Autodesk Inventor part; units mm, degrees
ref_plane "YZ Plane" through (0, 0, 0) normal (1, 0, 0) x (0, 1, 0)
ref_plane "XZ Plane" through (0, 0, 0) normal (0, 1, 0) x (-1, 0, 0)
ref_plane "XY Plane" through (0, 0, 0) normal (0, 0, 1) x (1, 0, 0)
sketch "Sketch1" plane through (0, 0, 0) normal (1, 0, 0) x (0, 1, 0)
  line L0 (0, 0) -> (0, -3.9878)
  line L1 (0, -3.9878) -> (0, -6.35)
  line L2 (0, -6.35) -> (3.175, -6.35)
  line L3 (3.175, -6.35) -> (3.175, -3.9878)
  line L4 (9.525, -3.9878) -> (9.525, -6.35)
  line L5 (9.525, -6.35) -> (12.7, -6.35)
  line L6 (12.7, -6.35) -> (12.7, -3.9878)
  line L7 (19.05, -3.9878) -> (19.05, -6.35)
  line L8 (19.05, -6.35) -> (22.225, -6.35)
  line L9 (22.225, -6.35) -> (22.225, -3.9878)
  line L10 (25.7937, 0) -> (0, 0)
  line L11 (51.5874, 0) -> (51.5874, -3.175)
  line L12 (51.5874, -3.175) -> (51.5874, -6.35)
  line L13 (51.5874, -6.35) -> (48.4124, -6.35)
  line L14 (48.4124, -6.35) -> (48.4124, -3.9878)
  line L15 (42.0624, -3.9878) -> (42.0624, -6.35)
  line L16 (42.0624, -6.35) -> (38.8874, -6.35)
  line L17 (38.8874, -6.35) -> (38.8874, -3.9878)
  line L18 (32.5374, -3.9878) -> (32.5374, -6.35)
  line L19 (32.5374, -6.35) -> (29.3624, -6.35)
  line L20 (29.3624, -6.35) -> (29.3624, -3.9878)
  line L21 (25.7937, 0) -> (51.5874, 0)
  line L22 (3.175, -3.9878) -> (9.525, -3.9878)
  line L23 (12.7, -3.9878) -> (19.05, -3.9878)
  line L24 (22.225, -3.9878) -> (29.3624, -3.9878)
  line L25 (32.5374, -3.9878) -> (38.8874, -3.9878)
  line L26 (42.0624, -3.9878) -> (48.4124, -3.9878)
  dimension "d1" = 3.9878
  dimension "d2" = 2.3622
  dimension "d3" = 3.175
  dimension "d5" = 3.175
  dimension "d7" = 3.175
revolve "Revolution1" add sketch "Sketch1" angle 360 about axis through (0, 25.7937, 0) along (0, 1, 0)
properties part number "Crankshaft Crank Cylinder"
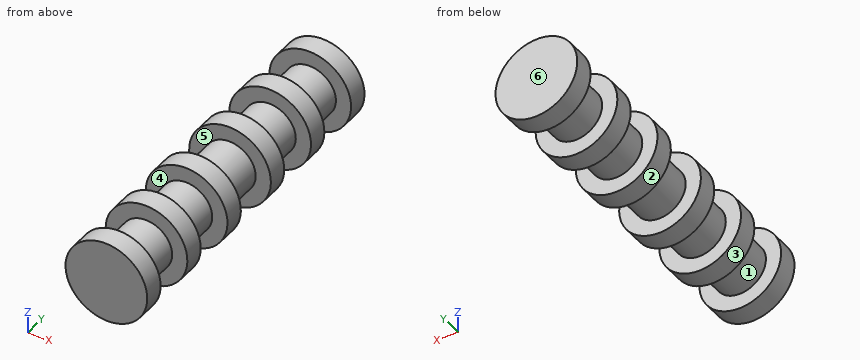
Verification items for the finished model (mm, model axes). Face numbers are marked on the shaded views. A direction names the side the tool comes from. Coordinates: 2 decimals unless noted, no trailing zeros. Loops run counter-clockwise (first coordinate to the right, second up) from the corner with the lowest first, then second, coordinate; pieces in that order, holes last. Notation, with made-up numbers: (87, -22.75) -> (138, -22.75) arc R7 cw to (138, -18.75) -> close; hole circle Ø11 at (19.5, 15.25). An arc over 180 degrees is marked (long way). Answer as CSV lines item,"result".
1) Tool access check on the marked faces 1 and 2. Record the directions out of +Z, -Z, +X, -X, +Y, -Y that give a thin tool (end or side, any length) a straight path to the whole face; none if there is none.
Found:
face 1,"none"
face 2,"+Y, -Y"
2) Depth check by flat-ended pin: pin 1 (1.5 mm diameter, centred on x = 2, y = 38.5, fed in from -Z); pin 2 (1.5 mm diameter, centred on y = 30, z = -4, fed in from +X); pin 3 (1.5 mm diameter, centred on x = -1.5, y = 24, fed in from -Z). Enter the tip coordinate at first touch or a pass-through.
Found:
pin 1,"stops at z = -6.2"
pin 2,"stops at x = 5.46"
pin 3,"stops at z = -3.92"
3) Thickness scan on L1, parallel to Y at x = 4, z = -1 (3 decimals); L2, parallel to Z at x = 0, y = 27; L3, parallel to Z at x = 1.75, y = 35. Record the ranges inside material, lowest first. Write a range as from..to.
Found:
L1,"y = 0..3.175, 9.525..12.7, 19.05..22.225, 29.362..32.537, 38.887..42.062, 48.412..51.587"
L2,"z = -3.99..3.99"
L3,"z = -3.58..3.58"
4) Cross-section at B-B, the plane z = -4.75. Record the cut outline in (x, y) (3 decimals), then the cut area to 3 significant figures.
Found:
outline,"(-4.214, 0) -> (4.214, 0) -> (4.214, 3.175) -> (-4.214, 3.175) -> close; (-4.214, 9.525) -> (4.214, 9.525) -> (4.214, 12.7) -> (-4.214, 12.7) -> close; (-4.214, 19.05) -> (4.214, 19.05) -> (4.214, 22.225) -> (-4.214, 22.225) -> close; (-4.214, 29.362) -> (4.214, 29.362) -> (4.214, 32.537) -> (-4.214, 32.537) -> close; (-4.214, 38.887) -> (4.214, 38.887) -> (4.214, 42.062) -> (-4.214, 42.062) -> close; (-4.214, 48.412) -> (4.214, 48.412) -> (4.214, 51.587) -> (-4.214, 51.587) -> close"
area,"161 mm2"
5) Cross-section at D-D, the plane y = 11.5. Record the cut outline in (x, z), then the cut area to 3 significant figures.
Found:
outline,"circle Ø12.7 at (0, 0)"
area,"127 mm2"
6) Cross-section at C-C, the plane y = 44. Record the cut outline in (x, z), then the cut area to 3 significant figures.
Found:
outline,"circle Ø7.98 at (0, 0)"
area,"50.0 mm2"
7) Release check for a two-part mould opening along Y. For the marked faces 3, 4, 5 and 6 record: +Y half, -Y half, draft (parallel to the pull), parting line (faces both ways), or undercut.
Found:
face 3,"draft"
face 4,"undercut"
face 5,"undercut"
face 6,"+Y half"
8) Cross-section at A-A, the plane x = -4.5. Record the cut outline in (y, z) (3 decimals).
Found:
outline,"(0, -4.48) -> (3.175, -4.48) -> (3.175, 4.48) -> (0, 4.48) -> close; (9.525, -4.48) -> (12.7, -4.48) -> (12.7, 4.48) -> (9.525, 4.48) -> close; (19.05, -4.48) -> (22.225, -4.48) -> (22.225, 4.48) -> (19.05, 4.48) -> close; (29.362, -4.48) -> (32.537, -4.48) -> (32.537, 4.48) -> (29.362, 4.48) -> close; (38.887, -4.48) -> (42.062, -4.48) -> (42.062, 4.48) -> (38.887, 4.48) -> close; (48.412, -4.48) -> (51.587, -4.48) -> (51.587, 4.48) -> (48.412, 4.48) -> close"
